For this review, take the finished solid that the model builds, in its own axes (mm). A direction names the side the tool comes from. Coordinates: 2 decimals unless noted, no trailing zeros. Loops run counter-clockwise (first coordinate to the right, second up) from the corner with the lowest first, then second, coordinate; pieces in that order, holes last. Notation, with made-up numbers: (-4, 1) -> (52, 1) arc R18 cw to (52, 20) -> close; hole circle Ø2 at (52, 62). An arc over 180 degrees is marked (long way). Answer in a Markdown table with one row per item.
from build123d import *

# Parameters (mm, degrees)
F1_DEPTH = 1
F3_R     = 0.375
F3_R_2   = 0.694729
F4_DEPTH = 25


with BuildPart() as f1:
    # F0 (on Front) → F1 (new body)
    with BuildSketch(Plane.XZ):
        with BuildLine():
            ThreePointArc((0, 6.145281), (0.292893, 5.438174), (1, 5.145281))
            Line((1, 5.145281), (9, 5.145281))
            Line((9, 5.145281), (9, -0.854719))
            ThreePointArc((9, -0.854719), (9.292893, -1.561826), (10, -1.854719))
            Line((10, -1.854719), (11, -1.854719))
            ThreePointArc((11, -1.854719), (11.707107, -1.561826), (12, -0.854719))
            Line((12, -0.854719), (12, 7.145281))
            ThreePointArc((12, 7.145281), (11.707107, 7.852388), (11, 8.145281))
            Line((11, 8.145281), (1, 8.145281))
            ThreePointArc((1, 8.145281), (0.292893, 7.852388), (0, 7.145281))
            Line((0, 7.145281), (0, 6.145281))
        make_face()
    extrude(amount=F1_DEPTH)

    # F3 (on face) → F4 (cut)
    with BuildSketch(Plane.XZ.offset(1)):
        with Locations((1, 7.345281)):
            Circle(F3_R)
        with Locations((1, 5.945281)):
            Circle(F3_R)
        with Locations((10.5, -0.354719)):
            Circle(F3_R_2)
    extrude(amount=-F4_DEPTH, mode=Mode.SUBTRACT)


solid = f1.part
Item 1: The part is to be moulded in two halves that separate along X. For faces 1 (the flat face through (7.2, -1, 5.4)), 2 (the cylindrical face through (9.285, -0.493, -1.554)), 3 (the cylindrical face through (9.806, -0.507, -0.324)), say which applies: +X half, -X half, draft (parallel to the pull), parting line (faces both ways), or undercut.
Worked answers:
| item | result |
|---|---|
| face 1 | draft |
| face 2 | -X half |
| face 3 | undercut |
Item 2: Take a section at D-D, the plane z = 0.5. State the section outline as (x, y) points.
Worked answers:
| item | result |
|---|---|
| outline | (9, -1) -> (12, -1) -> (12, 0) -> (9, 0) -> close |
Item 3: For L1, parallel to Z at x = 1, y = -0.65; L2, parallel to Z at x = 10.5, y = -0.1; L3, parallel to X at y = -0.2, z = 0.5, list the stretches that pass through material, from the lowest coordinate up.
Worked answers:
| item | result |
|---|---|
| L1 | 5.15 to 5.57, 6.32 to 6.97, 7.72 to 8.15 |
| L2 | -1.85 to -1.05, 0.34 to 8.15 |
| L3 | 9 to 12 |
Item 4: Take a section at B-B, the plane y = -0.8. State the section outline as (x, z) points (3 decimals), and give its area (3 significant figures).
Worked answers:
| item | result |
|---|---|
| outline | (0, 6.145) arc R1 ccw to (1, 5.145) -> (9, 5.145) -> (9, -0.855) arc R1 ccw to (10, -1.855) -> (11, -1.855) arc R1 ccw to (12, -0.855) -> (12, 7.145) arc R1 ccw to (11, 8.145) -> (1, 8.145) arc R1 ccw to (0, 7.145) -> close; hole circle Ø0.75 at (1, 5.945); hole circle Ø0.75 at (1, 7.345); hole circle Ø1.389 at (10.5, -0.355) |
| area | 53.5 mm² |
Item 5: Take a section at A-A, the plane x = 10.5. State the section outline as (y, z) points.
Worked answers:
| item | result |
|---|---|
| outline | (-1, -1.85) -> (0, -1.85) -> (0, -1.05) -> (-1, -1.05) -> close; (-1, 0.34) -> (0, 0.34) -> (0, 8.15) -> (-1, 8.15) -> close |
Item 6: Take a section at C-C, the plane x = 3.5. State the section outline as (y, z) points.
Worked answers:
| item | result |
|---|---|
| outline | (-1, 5.15) -> (0, 5.15) -> (0, 8.15) -> (-1, 8.15) -> close |
Item 7: For faces 4 (the flat face through (6.1, -0.5, 8.145)), 5 (the flat face through (9, -0.5, 2.2)), list the 3-axis set-ups (+Z, -Z, +X, -X, +Y, -Y) from which the entire face can be reached by the end or side of a thin tool; tool diameter is ignored.
Worked answers:
| item | result |
|---|---|
| face 4 | +Z, +X, -X, +Y, -Y |
| face 5 | -Z, -X, +Y, -Y |
